CAD build for the part. Positions are in the model's coordinates, mm. Face numbers are marked on the shaded views. A direction names the side the tool comes from. Round coordinates to 2 decimals unless told otherwise and drop trailing zeros. Write each loop counter-clockwise with the first axis right and the second up, starting at its lowest first coordinate (ties: lowest second). Pieces come first, ordered by that corner, then holes. Notation, with made-up numbers: M -8,37 L 38,37 A11 ccw 38,45 Z; hole C -28.75,-35 d1. An arc over 180 degrees is marked long. Write each question's results on one line, items separated by ' | '. Start each with the question number.
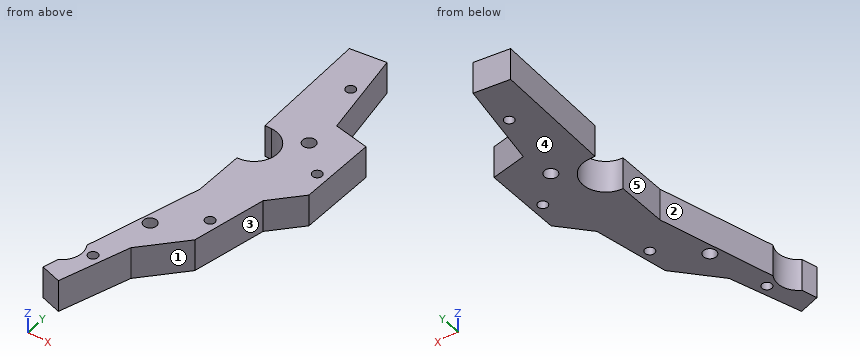
```python
from build123d import *

# Parameters (mm, degrees)
SKETCH1_R           = 0.75
SKETCH1_R_2         = 1
BOSS_EXTRUDE1_DEPTH = 5
SKETCH2_R           = 3.161990297
CUT_EXTRUDE3_DEPTH  = 6


with BuildPart() as part:
    # Sketch1 → Boss-Extrude1 (new body)
    with BuildSketch(Plane.XY):
        with BuildLine():
            Line((-54.335741925, 25.84189954), (-51.886829877, 12.115657968))
            Line((-51.886829877, 12.115657968), (-46.495560397, 11.056658606))
            Line((-46.495560397, 11.056658606), (-46.495560397, -0.8192261))
            Line((-46.495560397, -0.8192261), (-50.419003961, -5.159962771))
            Line((-50.419003961, -5.159962771), (-52.634709942, -16.439920489))
            Line((-52.634709942, -16.439920489), (-58.094962161, -22.48091908))
            Line((-58.094962161, -22.48091908), (-61.461861486, -33.112780309))
            Line((-61.461861486, -33.112780309), (-64.627062483, -32.110424007))
            Line((-64.627062483, -32.110424007), (-58.094962161, -8.109055729))
            Line((-58.094962161, -8.109055729), (-58.094962161, -0.397611229))
            ThreePointArc((-58.094962161, -0.397611229), (-54.514396766, 3.182954166), (-58.094962161, 6.763519562))
            Line((-58.094962161, 6.763519562), (-59.090495064, 6.763519562))
            Line((-59.090495064, 6.763519562), (-59.738806897, 25.184479172))
            Line((-59.738806897, 25.184479172), (-54.335741925, 25.84189954))
        make_face()
        with Locations((-54.792818894, 18.90647511)):
            Circle(SKETCH1_R, mode=Mode.SUBTRACT)
        with Locations((-48.15, 3.1)):
            Circle(SKETCH1_R, mode=Mode.SUBTRACT)
        with Locations((-53.399319926, -12.218458076)):
            Circle(SKETCH1_R, mode=Mode.SUBTRACT)
        with Locations((-60.980346807, -26.52714596)):
            Circle(SKETCH1_R, mode=Mode.SUBTRACT)
        with Locations((-52.634709942, 7.375968546)):
            Circle(SKETCH1_R_2, mode=Mode.SUBTRACT)
        with Locations((-59.090495064, -17.158775628)):
            Circle(SKETCH1_R_2, mode=Mode.SUBTRACT)
    extrude(amount=BOSS_EXTRUDE1_DEPTH)

    # Sketch2 → Cut-Extrude3 (cut, through all)
    with BuildSketch(Plane.XY):
        with Locations((-65.5, -27.039327647)):
            Circle(SKETCH2_R)
    extrude(amount=CUT_EXTRUDE3_DEPTH, mode=Mode.SUBTRACT)


solid = part.part
```
1) Saw through at C-C, the plane z = 4.5. Write the cut outline in (x, y).
2) Wall check: line 1 along Y through (x, z) = (-48.15, 2.55); line 2 along X through (y, z) = (-17, 4.2); line 3 along X through (y, z) = (7, 4.3). Give the ranges that are in metal, low to high. Write a range as from..to.
3) Pull direction Y, two halves, no side cores. Call the marked faces 3, 4 and 5: pulls with the +Y half, pulls with the -Y half, needs draft (parallel to the pull), parting line crosses it, or undercut.
4) Saw through at A-A, the plane x = -48.15. Write the cut outline in (y, z), plus the area to 3 significant figures.
5) 3-axis set-ups, long thin cutter, end or side, ignore diameter. For the marked faces 1 and 2: which of +Z, -Z, +X, -X, +Y, -Y reach the whole face in a straight line?
6) Saw through at B-B, the plane y = 3.1. Write the cut outline in (x, z), plus the area to 3 significant figures.
7) Saw through at D-D, the plane y = -7.5. Write the cut outline in (x, z), plus the area to 3 significant figures.
Filled sheet:
1) outline: M -64.63,-32.11 L -61.46,-33.11 L -58.09,-22.48 L -52.63,-16.44 L -50.42,-5.16 L -46.5,-0.82 L -46.5,11.06 L -51.89,12.12 L -54.34,25.84 L -59.74,25.18 L -59.09,6.76 L -58.09,6.76 A3.58 cw -58.09,-0.4 L -58.09,-8.11 L -62.8,-25.39 A3.16 cw -64.01,-29.83 Z; hole C -60.98,-26.53 d1.5; hole C -59.09,-17.16 d2; hole C -54.79,18.91 d1.5; hole C -53.4,-12.22 d1.5; hole C -52.63,7.38 d2; hole C -48.15,3.1 d1.5
2) line 1: y = -2.65..2.35, 3.85..11.38 | line 2: x = -60.51..-60.08, -58.1..-53.14 | line 3: x = -59.1..-53.56, -51.71..-46.5
3) face 3: pulls with the -Y half | face 4: needs draft | face 5: undercut
4) outline: M -2.65,0 L 2.35,0 L 2.35,5 L -2.65,5 Z; M 3.85,0 L 11.38,0 L 11.38,5 L 3.85,5 Z | area: 62.7 mm^2
5) face 1: +Z, -Z, +X, -Y | face 2: +Z, -Z, -X
6) outline: M -54.52,0 L -48.9,0 L -48.9,5 L -54.52,5 Z; M -47.4,0 L -46.5,0 L -46.5,5 L -47.4,5 Z | area: 32.6 mm^2
7) outline: M -58.09,0 L -50.88,0 L -50.88,5 L -58.09,5 Z | area: 36.1 mm^2
